The figure shows three views and two pictorial views of one solid part (mm, origin at its lowest corner). Answer the questions. A direction names the side the tool comes from. Give positions to 0.01 mm unless a question says otherwise; leave off trailing zeros. Write each loop counter-clockwise with the first axis right and the second up, starting at its lowest first coordinate (ties: lowest second). Pieces come first, ordered by that corner, then holes. Notation, with made-up numbers: (12.25, 17.25) -> (32.25, 17.25) arc R21 ccw to (32.25, 23.25) -> close; hole circle Ø6 at (38, 87). An arc over 180 degrees is marked (long way). Use a Markdown table: item, result.
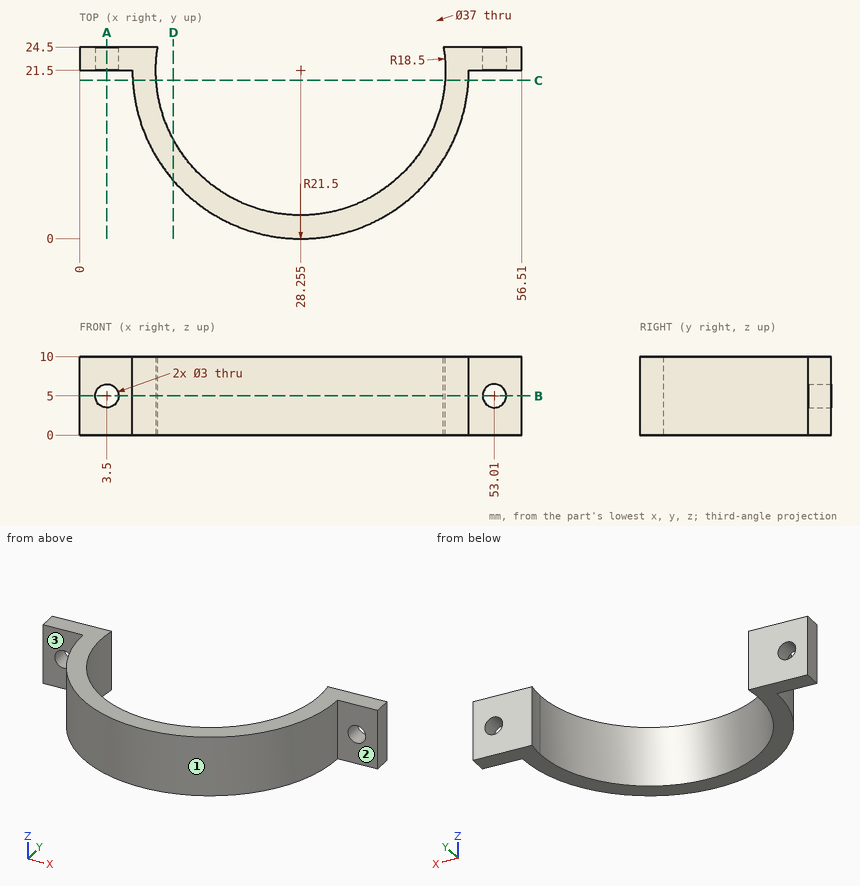
Item 1: Each of these flat-tipped pins is pushed along its axis until it touches: P1, Ø6, axis at y = 17, z = 6.5, coming from the -X side; P2, Ø3.5, axis at x = 53, z = 4, coming from the -Y side; P3, Ø2, axis at y = 3, z = 1, coming from the -X side (1 decimal); P4, Ø3, axis at x = 23.5, y = 4.5, coming from the +Z side. Where does it stop, or does it pass through?
Return value:
| item | result |
|---|---|
| P1 | x = 6.81 |
| P2 | y = 21.5 |
| P3 | x = 15.8 |
| P4 | z = 10 |
Item 2: A cutting plane is placed at D-D (x = 12). Give the vertices of the cut face in (y, z).
Return value:
| item | result |
|---|---|
| outline | (7.43, 0) -> (12.67, 0) -> (12.67, 10) -> (7.43, 10) -> close |
Item 3: A tool of negligible diameter and unlimited length cuts with its end or side. For the marked faces 1, 2 and 3, from which of +Z, -Z, +X, -X, +Y, -Y can it reach the whole face along a straight path? Write none if from no direction.
Return value:
| item | result |
|---|---|
| face 1 | +Z, -Z, -Y |
| face 2 | +Z, -Z, +X, -Y |
| face 3 | +Z, -Z, -X, -Y |
Item 4: A cutting plane is placed at A-A (x = 3.5). Give the vertices of the cut face in (y, z), then the cut area to 3 significant figures.
Return value:
| item | result |
|---|---|
| outline | (21.5, 0) -> (24.5, 0) -> (24.5, 3.5) -> (21.5, 3.5) -> close; (21.5, 6.5) -> (24.5, 6.5) -> (24.5, 10) -> (21.5, 10) -> close |
| area | 21.0 mm^2 |
Item 5: A cutting plane is placed at B-B (z = 5). Give the vertices of the cut face in (x, y) (1 decimal).
Return value:
| item | result |
|---|---|
| outline | (0, 21.5) -> (2, 21.5) -> (2, 24.5) -> (0, 24.5) -> close; (5, 21.5) -> (6.8, 21.5) arc R21.5 ccw to (49.8, 21.5) -> (51.5, 21.5) -> (51.5, 24.5) -> (46.5, 24.5) arc R18.5 cw (long way) to (10, 24.5) -> (5, 24.5) -> close; (54.5, 21.5) -> (56.5, 21.5) -> (56.5, 24.5) -> (54.5, 24.5) -> close |
Item 6: Straight lines are drawn through the part: line 1 along X through (y, z) = (21, 3); line 2 along Z through (x, y) = (3.5, 23.95); line 3 along Y through (x, z) = (50, 8.5). For each, find the intervals that lie inside material, in ascending order. Write a range as [from, to].
Return value:
| item | result |
|---|---|
| line 1 | [6.76, 9.76], [46.75, 49.75] |
| line 2 | [0, 3.5], [6.5, 10] |
| line 3 | [21.5, 24.5] |
Item 7: A cutting plane is placed at C-C (y = 20.25). Give the vertices of the cut face in (x, z).
Return value:
| item | result |
|---|---|
| outline | (6.79, 0) -> (9.8, 0) -> (9.8, 10) -> (6.79, 10) -> close; (46.71, 0) -> (49.72, 0) -> (49.72, 10) -> (46.71, 10) -> close |
